from build123d import *

# Parameters (mm, degrees)
CYLINDER025_R              = 1.5
CYLINDER025_DEPTH          = 4
CYLINDER020_R              = 2.1
CYLINDER020_DEPTH          = 9
CYLINDER019_R              = 4
CYLINDER019_DEPTH          = 12
CUT015_PLACEMENT_ANGLE     = 180
CYLINDER022_R              = 2.1
CYLINDER022_DEPTH          = 9
EXTRUDE005_DEPTH           = 3
EXTRUDE005_PLACEMENT_ANGLE = 270
CYLINDER021_R              = 2.1
CYLINDER021_DEPTH          = 9
BOX_W                      = 28
BOX_H                      = 46
BOX_DEPTH                  = 19
EXTRUDE009_DEPTH           = 21


with BuildPart() as ledhold001:
    # Cylinder025 → Cylinder025 (new body)
    with BuildSketch(Plane(origin=(-30, 0, 67), x_dir=(1, 0, 0), z_dir=(0, 0, 1))):
        Circle(CYLINDER025_R)
    extrude(amount=CYLINDER025_DEPTH)


with BuildPart() as insert006:
    # Cylinder020 → Cylinder020 (new body)
    with BuildSketch(Plane(origin=(5.5, -0.5, 1), x_dir=(1, 0, 0), z_dir=(0, 0, 1))):
        Circle(CYLINDER020_R)
    extrude(amount=CYLINDER020_DEPTH)


with BuildPart() as obj1:
    # Cylinder019 → Cylinder019 (new body)
    with BuildSketch(Plane(origin=(5.5, -0.5, -2), x_dir=(1, 0, 0), z_dir=(0, 0, 1))):
        Circle(CYLINDER019_R)
    extrude(amount=CYLINDER019_DEPTH)

    # Cut015: cut insert006
    add(insert006.part, mode=Mode.SUBTRACT)


with BuildPart() as obj1_1:
    # Cut015 placement: moved
    add(obj1.part.moved(Location((-34, -14.7, 66))).rotate(Axis((-34, -14.7, 66), (1, 0, 0)), CUT015_PLACEMENT_ANGLE))


with BuildPart() as obj2:
    # Clone006 base: copy of obj1
    add(obj1_1.part)


with BuildPart() as obj2_1:
    # Clone006 placement: moved
    add(obj2.part.moved(Location((0, 29.7, 0))))


with BuildPart() as insert008:
    # Cylinder022 → Cylinder022 (new body)
    with BuildSketch(Plane(origin=(-24, -25, 49), x_dir=(1, 0, 0), z_dir=(0, 0, 1))):
        Circle(CYLINDER022_R)
    extrude(amount=CYLINDER022_DEPTH)


with BuildPart() as usbextrude001:
    # Sketch005 → Extrude005 (new body)
    with BuildSketch(Plane(origin=(-2, -1, -5), x_dir=(1, 0, 0), z_dir=(0, -1, 0))):
        with BuildLine():
            ThreePointArc((16.408865, 14.741362), (13.786843, 12.11934), (16.408865, 9.497318))
            Line((16.408865, 9.497318), (23.664412, 9.497318))
            ThreePointArc((23.664412, 9.497318), (26.286434, 12.11934), (23.664412, 14.741362))
            Line((16.408865, 14.741362), (23.664412, 14.741362))
        make_face()
    extrude(amount=EXTRUDE005_DEPTH)


with BuildPart() as usbextrude001_1:
    # Extrude005 placement: moved
    add(usbextrude001.part.moved(Location((-36, 18, 54))).rotate(Axis((-36, 18, 54), (0, 0, 1)), EXTRUDE005_PLACEMENT_ANGLE))


with BuildPart() as fusion001:
    # Cylinder021 → Cylinder021 (new body)
    with BuildSketch(Plane(origin=(-24, 30, 49), x_dir=(1, 0, 0), z_dir=(0, 0, 1))):
        Circle(CYLINDER021_R)
    extrude(amount=CYLINDER021_DEPTH)

    # Fusion001: union insert008, usbExtrude001
    add(insert008.part)
    add(usbextrude001_1.part)


with BuildPart() as inner001:
    # Box → Box (new body)
    with BuildSketch(Plane(origin=(-38, -21, 49), x_dir=(1, 0, 0), z_dir=(0, 0, 1))):
        with Locations((14, 23)):
            Rectangle(BOX_W, BOX_H)
    extrude(amount=BOX_DEPTH)


with BuildPart() as obj3:
    # Sketch006 (on Face6 of Box) → Extrude009 (new body)
    with BuildSketch(Plane(origin=(-38, -21, 70), x_dir=(1, 0, 0), z_dir=(0, 0, 1))):
        with BuildLine():
            ThreePointArc((29.739196, 41.946692), (14.106739, 57.579149), (-1.525718, 41.946692))
            Line((-1.525718, 41.946692), (-1.525718, 4.775835))
            ThreePointArc((-1.525718, 4.775835), (14.106739, -10.856622), (29.739196, 4.775835))
            Line((29.739196, 41.946692), (29.739196, 4.775835))
        make_face()
    extrude(amount=-EXTRUDE009_DEPTH)

    # Cut016: cut inner001
    add(inner001.part, mode=Mode.SUBTRACT)

    # Cut017: cut Fusion001
    add(fusion001.part, mode=Mode.SUBTRACT)

    # Fusion002: union obj2, obj1
    add(obj2_1.part)
    add(obj1_1.part)

    # Cut019: cut ledHold001
    add(ledhold001.part, mode=Mode.SUBTRACT)


solid = obj3.part
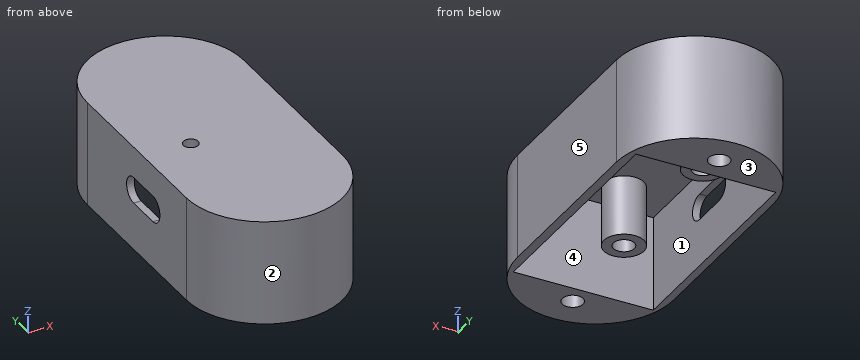
The listing builds one solid part. Answer for the finished solid, in the listing's coordinates (mm). Face numbers are marked on the shaded views. A direction names the side the tool comes from. Coordinates: 2 decimals unless noted, no trailing zeros. Write each loop counter-clockwise with the first axis right and the second up, starting at its lowest first coordinate (ties: lowest second). Pieces come first, ordered by that corner, then holes. Notation, with made-up numbers: M 60.5,3.25 L 96.5,3.25 A20 cw 96.5,31.25 Z; hole C 20.5,56 d6. An arc over 180 degrees is marked long. Put each result on its own line as item: value. Start each with the question number.
1. Consider line 1 (Y direction, x = -24, z = 53); line 2 (X direction, y = 0, z = 68.75); line 3 (X direction, y = 15.5, z = 62). Determine where each line is inside the solid, lowest interval first. Write a range as from..to.
2. A cutting plane is placed at B-B on y = 0. Write down the section's boundary in (x, z), then the cut area to 3 significant figures.
3. A cutting plane is placed at D-D on y = -14.2. Write down the section's boundary in (x, z).
4. A cutting plane is placed at A-A on z = 56.75. Write down the section's boundary in (x, y), then the cut area to 3 significant figures.
5. A cutting plane is placed at C-C on z = 52.25. Write down the section's boundary in (x, y), then the cut area to 3 significant figures.
6. Which of the six approach directions +Z, -Z, +X, -X, +Y, -Y give full straight-line access (tool end or side, diameter ignored) to the marked faces 4 and 5?
7. For a pull along X with two mould halves and no side action, classify the marked faces 1, 2 and 3 as pulls with the +X half, pulls with the -X half, needs draft (parallel to the pull), parting line crosses it, or undercut.
8. Flat-ended cylindrical pins translate along their axes: P1, Ø2.5, axis at x = -28, y = -15.5, coming from the -Z side; P2, Ø2, axis at y = -22, z = 53, coming from the +X side; P3, Ø4, axis at x = -21.5, z = 52, coming from the +Y side. Find the tip coordinate at first contact, or state that the pin passes through.
Resolved:
1. line 1: y = -31.86..-27.1, -22.9..-21, 25..27.9, 32.1..36.58
1. line 2: x = -39.53..-31.5, -28.5..-8.26
1. line 3: x = -39.53..-38, -32.5..-30.6, -26.4..-24.5, -10..-8.26
2. outline: M -39.53,49 L -38,49 L -38,58.5 L -39.53,58.5 Z; M -39.53,63.74 L -38,63.74 L -38,68 L -31.5,68 L -31.5,70 L -39.53,70 Z; M -28.5,68 L -10,68 L -10,49 L -8.26,49 L -8.26,70 L -28.5,70 Z
2. area: 111 mm2
3. outline: M -39.53,49 L -38,49 L -38,68 L -32.5,68 L -32.5,56 L -30.6,56 L -30.6,65 L -26.4,65 L -26.4,56 L -24.5,56 L -24.5,68 L -10,68 L -10,49 L -8.26,49 L -8.26,70 L -39.53,70 Z
4. outline: M -39.53,-16.22 A15.63 ccw -8.26,-16.22 L -8.26,20.95 A15.63 ccw -39.53,20.95 Z; C -28.5,-14.2 d8; C -28.5,15.5 d8; hole M -38,-21 L -10,-21 L -10,25 L -38,25 Z; hole C -28.5,-14.2 d4.2; hole C -28.5,15.5 d4.2; hole C -24,-25 d4.2; hole C -24,30 d4.2
4. area: 687 mm2
5. outline: M -39.53,-16.22 A15.63 ccw -8.26,-16.22 L -8.26,20.95 A15.63 ccw -39.53,20.95 Z; hole M -38,-21 L -10,-21 L -10,25 L -38,25 Z; hole C -24,-25 d4.2; hole C -24,30 d4.2
5. area: 614 mm2
6. face 4: -Z
6. face 5: +Z, -Z, +X, +Y, -Y
7. face 1: undercut
7. face 2: parting line crosses it
7. face 3: needs draft
8. P1: stops at z = 56
8. P2: stops at x = -9.01
8. P3: stops at y = 36.57
